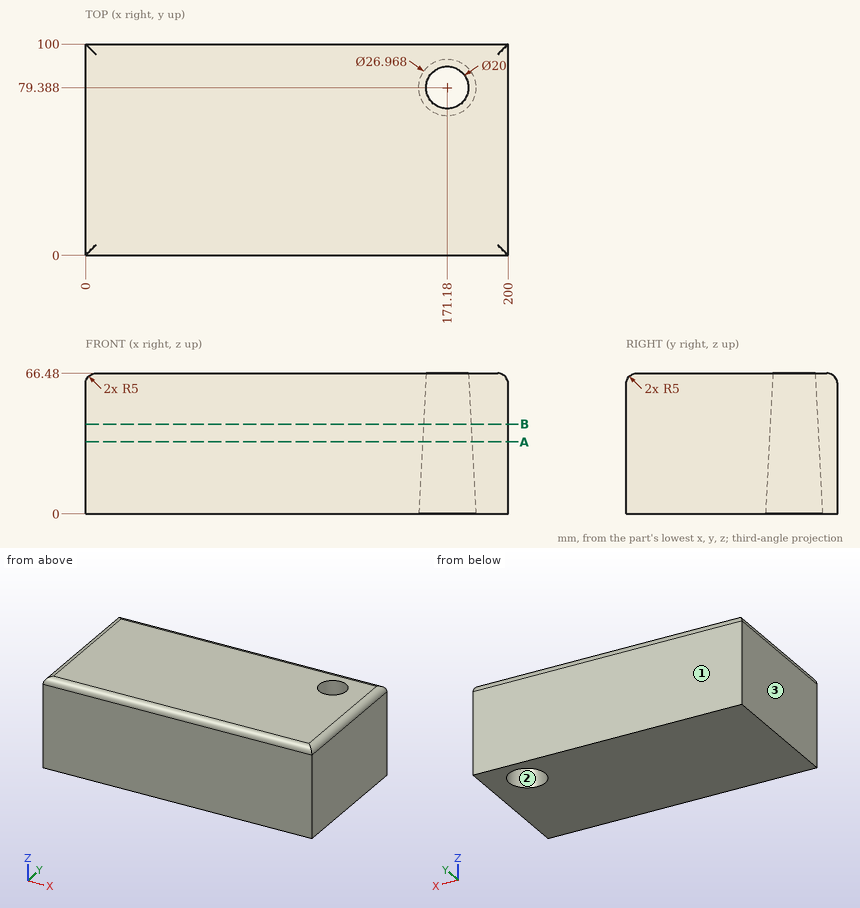
Input: dimensioned drawing with shaded views. Units: mm. Origin: part minimum x, y, z. Round coordinates to 2 decimals unless told otherwise and drop trailing zeros. Loops run counter-clockwise (first coordinate to the right, second up) from the corner with the lowest first, then second, coordinate; pieces in that order, holes last.
1) Section query B-B on z = 42.5. Return the cut outline in (x, y), plus the area to 3 significant figures.
Ans:
outline: (0, 0) - (200, 0) - (200, 100) - (0, 100) - close; hole circle Ø22.51 at (171.18, 79.39)
area: 19,600 mm2
2) Pull-direction query (X, two-part tool) for the marked faces 1, 2 and 3; classes: released by +X, released by -X, zero draft, split by the parting line, or undercut.
Ans:
face 1: zero draft
face 2: undercut
face 3: released by -X
3) Material intervals for line 1 (X direction, y = 77, z = 10); line 2 (X direction, y = 77.5, z = 18); line 3 (X direction, y = 22, z = 63.5) (1 decimal), sorted ascending.
Ans:
line 1: x = 0 to 158.44, 183.92 to 200
line 2: x = 0 to 158.78, 183.58 to 200
line 3: x = 0.4 to 199.6
4) Section query A-A on z = 34. Return the cut outline in (x, y) (1 decimal).
Ans:
outline: (0, 0) - (200, 0) - (200, 100) - (0, 100) - close; hole circle Ø23.4 at (171.2, 79.4)
